CAD build for the part. Positions are in the model's coordinates, mm. A direction names the side the tool comes from. Give positions to 0.01 mm unless a question says otherwise; leave off trailing zeros. Loops run counter-clockwise (first coordinate to the right, second up) from the corner with the lowest first, then second, coordinate; pieces in that order, holes last. Notation, with made-up numbers: M -36.5,52.5 L 11.5,52.5 A20 cw 11.5,87.5 Z; hole C 13.25,21.5 d4. An arc over 180 degrees is marked long. Answer as CSV lines item,"result".
```python
from build123d import *

# Parameters (mm, degrees)
F1_DEPTH = 150
F2_R     = 22.5
F3_DEPTH = 50
F4_R     = 22.5
F5_DEPTH = 50


with BuildPart() as f1:
    # F0 (on Front) → F1 (new body, symmetric)
    with BuildSketch(Plane.XZ):
        with BuildLine():
            ThreePointArc((0, 70), (20.5025253169, 20.5025253169), (70, 0))
            Line((70, 0), (1020, 0))
            ThreePointArc((1020, 0), (1069.4974746831, 20.5025253169), (1090, 70))
            Line((1090, 70), (1090, 300))
            Line((1090, 300), (1040, 300))
            Line((1040, 300), (1040, 70))
            ThreePointArc((1040, 70), (1034.1421356237, 55.8578643763), (1020, 50))
            Line((1020, 50), (70, 50))
            ThreePointArc((70, 50), (55.8578643763, 55.8578643763), (50, 70))
            Line((50, 70), (50, 500))
            Line((50, 500), (0, 500))
            Line((0, 500), (0, 70))
        make_face()
    extrude(amount=F1_DEPTH, both=True)

    # F2 (on face) → F3 (cut, through all)
    with BuildSketch(Plane.YZ.offset(1090)):
        with Locations((0, 200)):
            Circle(F2_R)
    extrude(amount=-F3_DEPTH, mode=Mode.SUBTRACT)

    # F4 (on face) → F5 (cut, through all)
    with BuildSketch(Plane(origin=(0, 0, 0), x_dir=(0, -1, 0), z_dir=(-1, 0, 0))):
        with Locations((0, 400)):
            Circle(F4_R)
    extrude(amount=-F5_DEPTH, mode=Mode.SUBTRACT)


solid = f1.part
```
Q1. Pin check, flat tip, straight feed: P1, Ø1, axis at x = 368, y = 41, coming from the +Z side. Stop position of the tip, or through.
Solution:
P1,"stops at z = 50"
Q2. Which spindle directions (+Z, -Z, +X, -X, +Y, -Y) get a long thin tool onto all of the face, cutting with end or side? Do faces 1 (the flat face through (1065, -2, 300)), 2 (the cylindrical face through (1065.35, -2.93, 222.31)), 3 (the flat face through (1040, -2, 161)). Say none if no direction does.
Solution:
face 1,"+Z, +X, +Y, -Y"
face 2,"+X"
face 3,"+Z, +Y, -Y"
Q3. Cut at D-D (y = 71.5). Write the cut outline in (x, z), and give its area (3 significant figures).
Solution:
outline,"M 0,70 A70 ccw 70,0 L 1020,0 A70 ccw 1090,70 L 1090,300 L 1040,300 L 1040,70 A20 cw 1020,50 L 70,50 A20 cw 50,70 L 50,500 L 0,500 Z"
area,"87,600 mm²"
Q4. Cut at C-C (z = 200). Write the cut outline in (x, y), and give its area (4 significant figures).
Solution:
outline,"M 0,-150 L 50,-150 L 50,150 L 0,150 Z; M 1040,-150 L 1090,-150 L 1090,-22.5 L 1040,-22.5 Z; M 1040,22.5 L 1090,22.5 L 1090,150 L 1040,150 Z"
area,"27,750 mm²"
Q5. Cut at A-A (z = 82). Write the cut outline in (x, y), and give its area (3 significant figures).
Solution:
outline,"M 0,-150 L 50,-150 L 50,150 L 0,150 Z; M 1040,-150 L 1090,-150 L 1090,150 L 1040,150 Z"
area,"30,000 mm²"
Q6. Wall check: line 1 (X direction, y = 129, z = 268); line 2 (Z direction, x = 18.5, y = 0); line 3 (Z direction, x = 147, y = 82.5). Give the ranges that are in metal, low to high. Write a range as [from, to].
Solution:
line 1,"x = [0, 50], [1040, 1090]"
line 2,"z = [22.59, 377.5], [422.5, 500]"
line 3,"z = [0, 50]"
Q7. Cut at B-B (y = 0). Write the cut outline in (x, z).
Solution:
outline,"M 0,70 A70 ccw 70,0 L 1020,0 A70 ccw 1090,70 L 1090,177.5 L 1040,177.5 L 1040,70 A20 cw 1020,50 L 70,50 A20 cw 50,70 L 50,377.5 L 0,377.5 Z; M 0,422.5 L 50,422.5 L 50,500 L 0,500 Z; M 1040,222.5 L 1090,222.5 L 1090,300 L 1040,300 Z"
Q8. Mould opens along X. For faces 4 (the cylindrical face through (24.65, -12.1, 418.97)), 5 (the flat face through (50, -2, 282)), 6 (the flat face through (1090, -2, 158)), 7 (the cylindrical face through (56.014, -2.1, 55.703)) say: released by +X, released by -X, zero draft, split by the parting line, or undercut.
Solution:
face 4,"zero draft"
face 5,"undercut"
face 6,"released by +X"
face 7,"undercut"
